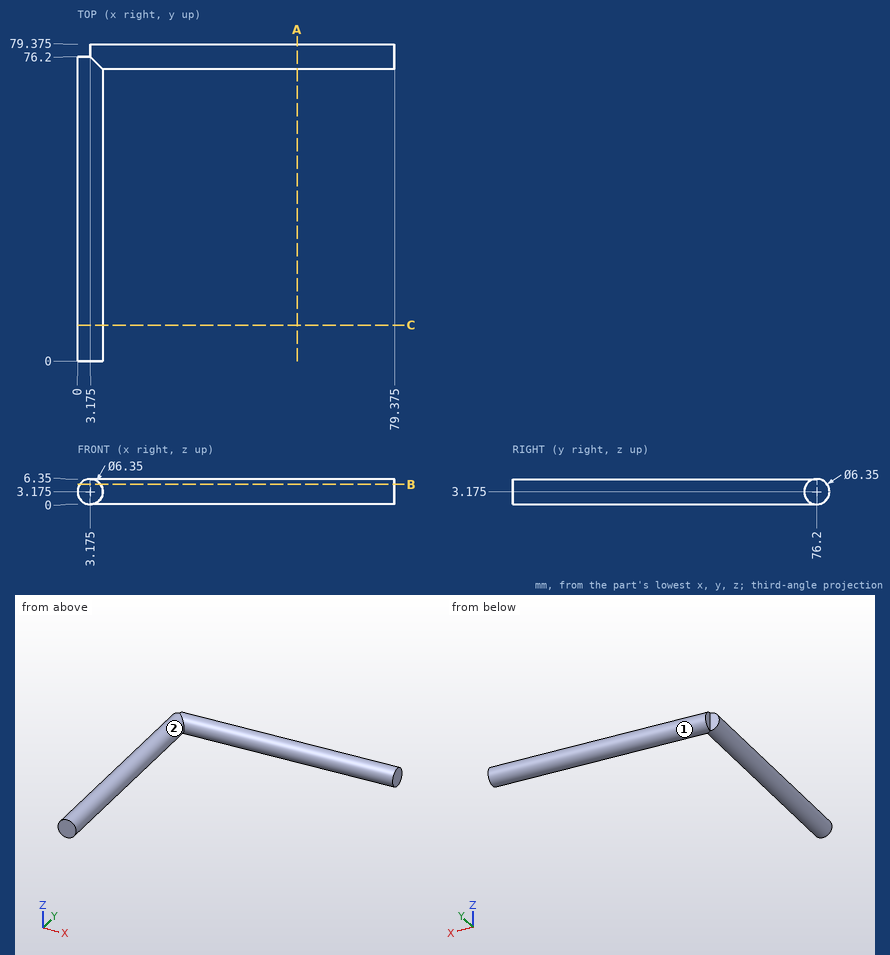
Input: dimensioned drawing with shaded views. Units: mm. Origin: part minimum x, y, z. Round coordinates to 2 decimals unless told otherwise and drop trailing zeros. Order: outer loops, then holes, each group sorted by start corner. A loop starts at its lowest first (then second) coordinate and runs counter-clockwise, first axis right, second up. Notation, with made-up numbers: (81, 68.25) -> (132, 68.25) arc R21 cw to (132, 101.25) -> close; hole circle Ø5 at (-14.75, -36). An arc over 180 degrees is marked (long way). Put each result on its own line as item: value. Start each with the question number.
Q1. Line query: probe 1 along Y at (x, z) = (9, 3.5); probe 2 along X at (y, z) = (18.5, 3.25); probe 3 along X at (y, z) = (59.5, 4). Output: solid intervals per line, ascending.
Q2. Pull-direction query (Y, two-part tool) for the marked faces 1 and 2; classes: +Y half, -Y half, draft (parallel to the pull), parting line (faces both ways), or undercut.
Q3. Section A-A on x = 55. Return the cut outline in (y, z) (3 decimals).
Q4. Section C-C on y = 9. Return the cut outline in (x, z) (3 decimals).
Q5. First-contact query: pin 1 (1 mm diameter, centred on y = 36, z = 2.5, fed in from -X); pin 2 (1.6 mm diameter, centred on y = 78, z = 3, fed in from -X) (3 decimals); pin 3 (1.5 mm diameter, centred on x = 23.5, z = 3, fed in from +Y) (3 decimals); pin 4 (1 mm diameter, centred on x = 1, z = 3.5, fed in from +Y). Flat tips, straight axial feed; report the tip coordinate or a pass-through.
Q6. Section B-B on z = 5. Return the cut outline in (x, y) (3 decimals).
Ans:
1. probe 1: y = 73.04 to 79.36
1. probe 2: x = 0 to 6.35
1. probe 3: x = 0.11 to 6.24
2. face 1: parting line
2. face 2: draft
3. outline: circle Ø6.35 at (76.2, 3.175)
4. outline: circle Ø6.35 at (3.175, 3.175)
5. pin 1: stops at x = 0
5. pin 2: stops at x = 3.175
5. pin 3: stops at y = 79.375
5. pin 4: stops at y = 76.2
6. outline: (0.577, 0) -> (5.773, 0) -> (5.773, 73.602) -> (79.375, 73.602) -> (79.375, 78.798) -> (3.175, 78.798) -> (3.175, 76.2) -> (0.577, 76.2) -> close
